Here's how the part is built. I have some questions about the finished solid (model axes, mm). Face numbers are marked on the shaded views. A direction names the side the tool comes from. Round coordinates to 2 decimals unless told otherwise and drop trailing zeros. Loops run counter-clockwise (first coordinate to the right, second up) from the corner with the lowest first, then second, coordinate; pieces in that order, holes last. Notation, with made-up numbers: M 68.25,-26 L 73.25,-26 A15 ccw 73.25,-5 Z; hole C 16,4.25 d9. An arc over 180 degrees is marked long. Put each result on its own line as item: value. Start each with the question number.
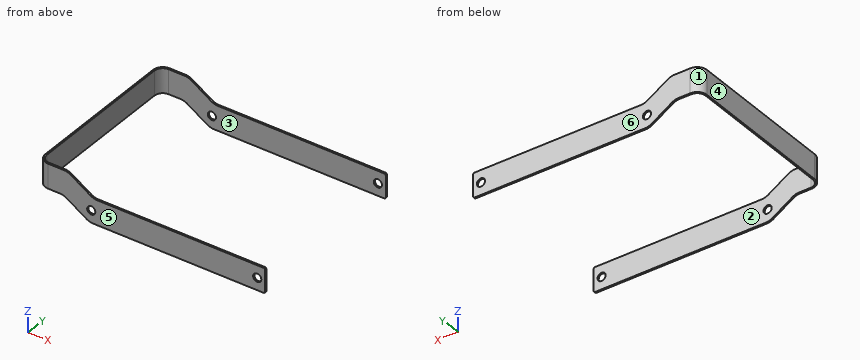
```python
from build123d import *

# Parameters (mm, degrees)
SKETCH002_R  = 2.5
PAD001_DEPTH = 51.75
PAD_DEPTH    = 30


with BuildPart() as face_body:
    # Sketch002 → Pad001 (new body, symmetric)
    with BuildSketch(Plane.XZ):
        with BuildLine():
            Line((-57.529972, 0), (47.470028, 0))
            ThreePointArc((47.470028, 0), (48.177135, 0.292893), (48.470028, 1))
            Line((48.470028, 14), (48.470028, 1))
            ThreePointArc((48.470028, 14), (48.177135, 14.707107), (47.470028, 15))
            Line((-55.029972, 15), (47.470028, 15))
            ThreePointArc((-58.176393, 16), (-56.645942, 15.365461), (-55.029972, 15))
            Line((-70.88355, 24.00071), (-58.176393, 16))
            ThreePointArc((-70.88355, 24.00071), (-72.414001, 24.635249), (-74.029972, 25.00071))
            Line((-89.029972, 25), (-74.029972, 25.00071))
            Line((-90.529972, 25), (-89.029972, 25))
            Line((-90.529972, 25), (-90.529972, 10))
            Line((-90.529972, 10), (-89.029972, 10))
            Line((-89.029972, 10), (-76.529972, 10.000632))
            ThreePointArc((-73.383499, 9.000791), (-74.904353, 9.665557), (-76.529972, 10.000632))
            Line((-73.383499, 9.000791), (-60.676393, 1))
            ThreePointArc((-60.676393, 1), (-59.145942, 0.365461), (-57.529972, 0))
        make_face()
        with Locations((-58.005918, 7.5)):
            Circle(SKETCH002_R, mode=Mode.SUBTRACT)
        with Locations((43.594082, 7.5)):
            Circle(SKETCH002_R, mode=Mode.SUBTRACT)
    extrude(amount=PAD001_DEPTH, both=True)


with BuildPart() as base_body:
    # Sketch001 → Pad (new body)
    with BuildSketch(Plane.XY):
        with BuildLine():
            Line((-89.459922, 45.75), (-89.459922, -45.75))
            ThreePointArc((-89.459922, -45.75), (-87.995456, -49.285534), (-84.459922, -50.75))
            Line((48.594082, -50.75), (-84.459922, -50.75))
            Line((48.594082, -50.75), (48.594082, -51.75))
            Line((-84.459922, -51.75), (48.594082, -51.75))
            ThreePointArc((-90.459922, -45.75), (-88.702563, -49.992641), (-84.459922, -51.75))
            Line((-90.459922, 45.750008), (-90.459922, -45.75))
            ThreePointArc((-84.459922, 51.75), (-88.70256, 49.992644), (-90.459922, 45.750008))
            Line((-84.459922, 51.75), (48.594082, 51.75))
            Line((48.594082, 50.75), (48.594082, 51.75))
            Line((48.594082, 50.75), (-84.459922, 50.75))
            ThreePointArc((-84.459922, 50.75), (-87.995456, 49.285534), (-89.459922, 45.75))
        make_face()
    extrude(amount=PAD_DEPTH)

    # Boolean: intersect Face.Body
    add(face_body.part, mode=Mode.INTERSECT)


solid = base_body.part
```
1) Suppose I cut it at C-C (z = 19). Write out the boundary of the cut face in (x, y), plus the area to 3 significant figures.
2) If I drill on probe 1 along Y at (x, z) = (-13, 10.5); probe 2 along X at (y, z) = (-51.4, 7.5); probe 3 along X at (y, z) = (-5, 12.5), over which ranges is the centre line in solid material (lowest first)? Write a range as from..to.
3) Suppose I cut it at A-A (x = 38.5). Write out the boundary of the cut face in (y, z).
4) I'm going to push flat-ended pins straight in: P1, Ø2, axis at x = -84, y = -50.5, coming from the +Z side; P2, Ø0.5, axis at x = -22.5, y = 51, coming from the +Z side; P3, Ø4.5, axis at x = -81.5, y = 49.5, coming from the -Z side; P4, Ø7.5, axis at y = -15.5, z = 17.5, coming from the +X side. Where does each tip first touch, or does it pass through?
5) On a 3-axis mill with a long thin cutter (end or side, diameter ignored), from which of +Z, -Z, +X, -X, +Y, -Y can I reach the whole of each face in a straight line? I mean the marked faces 1 and 2. Say none if no direction works.
6) Suppose I cut it at B-B (z = 7.5). Write out the boundary of the cut face in (x, y).
7) Suppose I cut it at D-D (y = 6). Write out the boundary of the cut face in (x, z), plus the area to 3 significant figures.
8) If we mould it in two halves opening along Y, with no side actions, what happens to the marked faces 3, 4, 5 and 6? For each: pulls with the +Y half, pulls with the -Y half, needs draft (parallel to the pull), parting line crosses it, or undercut.
Results are:
1. outline: M -90.46,-45.75 A6 ccw -84.46,-51.75 L -62.94,-51.75 L -62.94,-50.75 L -84.46,-50.75 A5 cw -89.46,-45.75 L -89.46,45.75 A5 cw -84.46,50.75 L -62.94,50.75 L -62.94,51.75 L -84.46,51.75 A6 ccw -90.46,45.75 Z
1. area: 152 mm²
2. probe 1: -51.75..-50.75, 50.75..51.75
2. probe 2: -71..-60.51, -55.51..41.09, 46.09..48.47
2. probe 3: -90.46..-89.46
3. outline: M -51.75,0 L -50.75,0 L -50.75,15 L -51.75,15 Z; M 50.75,0 L 51.75,0 L 51.75,15 L 50.75,15 Z
4. P1: z = 25
4. P2: z = 15
4. P3: z = 10
4. P4: x = -89.46
5. face 1: +Z, -Z, -X, +Y
5. face 2: +Z, -Z, +X
6. outline: M -71,-51.75 L -60.51,-51.75 L -60.51,-50.75 L -71,-50.75 Z; M -71,50.75 L -60.51,50.75 L -60.51,51.75 L -71,51.75 Z; M -55.51,-51.75 L 41.09,-51.75 L 41.09,-50.75 L -55.51,-50.75 Z; M -55.51,50.75 L 41.09,50.75 L 41.09,51.75 L -55.51,51.75 Z; M 46.09,-51.75 L 48.47,-51.75 L 48.47,-50.75 L 46.09,-50.75 Z; M 46.09,50.75 L 48.47,50.75 L 48.47,51.75 L 46.09,51.75 Z
7. outline: M -90.46,10 L -89.46,10 L -89.46,25 L -90.46,25 Z
7. area: 15.0 mm²
8. face 3: undercut
8. face 4: needs draft
8. face 5: pulls with the -Y half
8. face 6: pulls with the +Y half
